```python
from build123d import *

# Parameters (mm, degrees)
CYLINDER001_R     = 1.6
CYLINDER001_DEPTH = 10
CYLINDER_R        = 3
CYLINDER_DEPTH    = 8


with BuildPart() as cylinder001:
    # Cylinder001 → Cylinder001 (new body)
    with BuildSketch(Plane.XY.offset(-1)):
        Circle(CYLINDER001_R)
    extrude(amount=CYLINDER001_DEPTH)


with BuildPart() as cut:
    # Cylinder → Cylinder (new body)
    with BuildSketch(Plane.XY):
        Circle(CYLINDER_R)
    extrude(amount=CYLINDER_DEPTH)

    # Cut: cut Cylinder001
    add(cylinder001.part, mode=Mode.SUBTRACT)


solid = cut.part
```
Work out the finished part from the listing and answer in its coordinate system (mm). Round coordinates to 2 decimals unless told otherwise and drop trailing zeros. Write each loop counter-clockwise with the first axis right and the second up, starting at its lowest first coordinate (ties: lowest second). Pieces come first, ordered by that corner, then holes.
1) A cutting plane is placed at C-C on z = 1.75. Determine the outline of the cut face in (x, y), and give its area (3 significant figures).
2) A cutting plane is placed at A-A on y = 0. Determine the outline of the cut face in (x, z).
3) A cutting plane is placed at D-D on x = -1.9. Determine the outline of the cut face in (y, z), and give its area (3 significant figures).
4) Consider probe 1 along Y at (x, z) = (0, 5.5); probe 2 along X at (y, z) = (-1, 2.25); probe 3 along X at (y, z) = (-0.3, 0.75). Determine where each line is inside the solid, lowest interval first.
5) Flat-ended cylindrical pins translate along their axes: P1, Ø3.5, axis at x = 0, y = 0, coming from the +Z side; P2, Ø1.5, axis at y = -2.5, z = 1, coming from the +X side; P3, Ø1, axis at x = -1, z = 2, coming from the -Y side. Find the tip coordinate at first contact, or state that the pin passes through.
6) Determine the mould class of faces 1 (the face through (1.3, -1.3, 8)), 2 (the face through (-3, 0, 4)), 3 (the face through (-1.27, -0.97, 3.94)) for opening direction Y: pulls with the +Y half, pulls with the -Y half, needs draft (parallel to the pull), parting line crosses it, or undercut.
Entries:
1. outline: circle Ø6 at (0, 0); hole circle Ø3.2 at (0, 0)
1. area: 20.2 mm2
2. outline: (-3, 0) - (-1.6, 0) - (-1.6, 8) - (-3, 8) - close; (1.6, 0) - (3, 0) - (3, 8) - (1.6, 8) - close
3. outline: (-2.32, 0) - (2.32, 0) - (2.32, 8) - (-2.32, 8) - close
3. area: 37.1 mm2
4. probe 1: y = -3 to -1.6, 1.6 to 3
4. probe 2: x = -2.83 to -1.25, 1.25 to 2.83
4. probe 3: x = -2.98 to -1.57, 1.57 to 2.98
5. P1: stops at z = 8
5. P2: stops at x = 2.44
5. P3: stops at y = -2.96
6. face 1: needs draft
6. face 2: parting line crosses it
6. face 3: undercut
